from build123d import *

# Parameters (mm, degrees)
BOSS_EXTRUDE1_DEPTH = 6.35


with BuildPart() as part:
    # Sketch1 → Boss-Extrude1 (new body)
    with BuildSketch(Plane.XY):
        Polygon((27.78125, 44.45), (31.75, 44.45), (31.75, 50.8), (44.45, 50.8), (44.45, 44.45), (50.8, 44.45), (50.8, 6.35), (44.45, 6.35), (44.45, 0), (31.75, 0), (31.75, 6.35), (27.78125, 6.35), (27.78125, 11.1125), (30.1625, 11.1125), (30.1625, 14.2875), (27.78125, 14.2875), (27.78125, 17.4625), (23.01875, 17.4625), (23.01875, 14.2875), (20.6375, 14.2875), (20.6375, 11.1125), (23.01875, 11.1125), (23.01875, 6.35), (19.05, 6.35), (19.05, 0), (6.35, 0), (6.35, 6.35), (0, 6.35), (0, 44.45), (6.35, 44.45), (6.35, 50.8), (19.05, 50.8), (19.05, 44.45), (23.01875, 44.45), (23.01875, 39.6875), (20.6375, 39.6875), (20.6375, 36.5125), (23.01875, 36.5125), (23.01875, 33.3375), (27.78125, 33.3375), (27.78125, 36.5125), (30.1625, 36.5125), (30.1625, 39.6875), (27.78125, 39.6875), align=None)
    extrude(amount=BOSS_EXTRUDE1_DEPTH)


solid = part.part
Geometry check sheet. Reference: the model listing, model coordinates, mm. A direction names the side the tool comes from. Round coordinates to 2 decimals unless told otherwise and drop trailing zeros. Write each loop counter-clockwise with the first axis right and the second up, starting at its lowest first coordinate (ties: lowest second). Pieces come first, ordered by that corner, then holes.
Item 1: Access from +Z, -Z, +X, -X, +Y, -Y to the whole of each face (thin tool, end or side, straight path). Record for faces 1 (the face through (23.019, 35, 3)), 2 (the face through (19.05, 3, 3)), 3 (the face through (6.35, 48, 3)), 4 (the face through (29, 14.288, 3)).
Determined:
face 1: +Z, -Z, +Y
face 2: +Z, -Z, -Y
face 3: +Z, -Z, -X, +Y
face 4: +Z, -Z
Item 2: Section check C-C (y = 47). Record the boundary of the cut face in (x, z), plus the area to 3 significant figures.
Determined:
outline: (6.35, 0) - (19.05, 0) - (19.05, 6.35) - (6.35, 6.35) - close; (31.75, 0) - (44.45, 0) - (44.45, 6.35) - (31.75, 6.35) - close
area: 161 mm2
Item 3: Go/stop test with flat-tipped pins: pin 1 Ø1.2 at (x, z) = (20, 3.5) entering from -Y; pin 2 Ø1.2 at (x, z) = (30, 4) entering from +Y; pin 3 Ø2 at (x, y) = (33, 30) entering from -Z; pin 4 Ø1.9 at (y, z) = (48, 3) entering from -X. Record where each tip stops, or that it passes through.
Determined:
pin 1: stops at y = 6.35
pin 2: stops at y = 44.45
pin 3: stops at z = 0
pin 4: stops at x = 6.35
Item 4: Section check B-B (x = 29). Record the boundary of the cut face in (y, z), plus the area to 3 significant figures.
Determined:
outline: (6.35, 0) - (11.11, 0) - (11.11, 6.35) - (6.35, 6.35) - close; (14.29, 0) - (36.51, 0) - (36.51, 6.35) - (14.29, 6.35) - close; (39.69, 0) - (44.45, 0) - (44.45, 6.35) - (39.69, 6.35) - close
area: 202 mm2
Item 5: Mould release check, pull along X, two halves, no side actions. Record for faces 5 (the face through (25, 33.338, 3)), 6 (the face through (13, 50.8, 3)), 7 (the face through (6.35, 3, 3)), 8 (the face through (50.8, 26, 3)): +X half, -X half, draft (parallel to the pull), parting line (faces both ways), or undercut.
Determined:
face 5: undercut
face 6: draft
face 7: -X half
face 8: +X half
Item 6: Section check A-A (y = 7.5). Record the boundary of the cut face in (x, z), plus the area to 3 significant figures.
Determined:
outline: (0, 0) - (23.02, 0) - (23.02, 6.35) - (0, 6.35) - close; (27.78, 0) - (50.8, 0) - (50.8, 6.35) - (27.78, 6.35) - close
area: 292 mm2
Item 7: Material ranges on line 1 along Y through (x, z) = (21, 2.5); line 2 along X through (y, z) = (45.5, 0.75); line 3 along Y through (x, z) = (45, 3.5), recorded low to high.
Determined:
line 1: y = 6.35 to 11.11, 14.29 to 36.51, 39.69 to 44.45
line 2: x = 6.35 to 19.05, 31.75 to 44.45
line 3: y = 6.35 to 44.45
